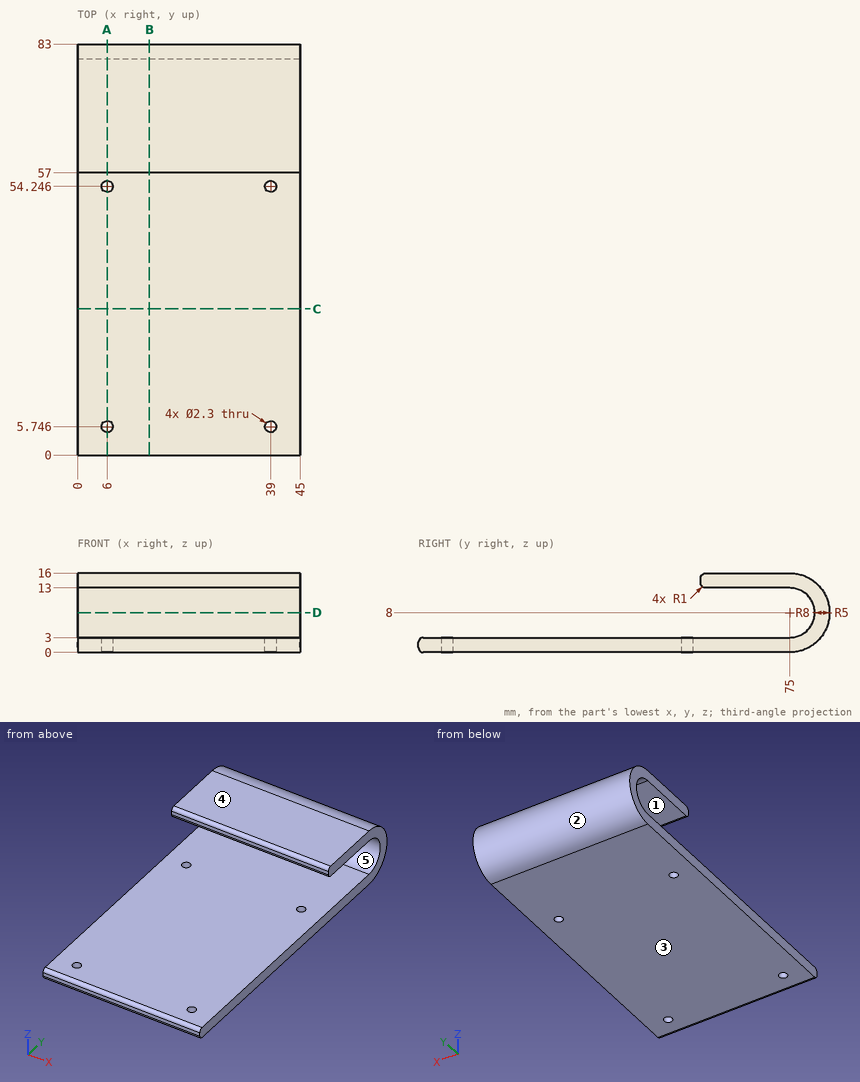
Can you work these out from the drawing? Everything is in mm from the part's minimum corner. A direction names the side the tool comes from. Coordinates: 2 decimals unless noted, no trailing zeros. Loops run counter-clockwise (first coordinate to the right, second up) from the corner with the lowest first, then second, coordinate; pieces in that order, holes last. Notation, with made-up numbers: (-38.75, 53) - (-31.75, 53) arc R11 ccw to (-31.75, 64) - close; hole circle Ø6 at (83, 40.5). An arc over 180 degrees is marked (long way). Use a Markdown table: item, result.
Item 1: I want a section at C-C on y = 29.5. Please give me the cut outline in (x, z), and give its area (3 significant figures).
Numbers:
| item | result |
|---|---|
| outline | (0, 0) - (45, 0) - (45, 3) - (0, 3) - close |
| area | 135 mm2 |
Item 2: I want a section at D-D on z = 8. Please give me the cut outline in (x, y), and give its area (3 significant figures).
Numbers:
| item | result |
|---|---|
| outline | (0, 80) - (45, 80) - (45, 83) - (0, 83) - close |
| area | 135 mm2 |
Item 3: I want a section at A-A on x = 6. Please give me the cut outline in (y, z), and give its area (3 significant figures).
Numbers:
| item | result |
|---|---|
| outline | (0, 1) arc R1 ccw to (1, 0) - (4.6, 0) - (4.6, 3) - (1, 3) arc R1 ccw to (0, 2) - close; (6.9, 0) - (53.1, 0) - (53.1, 3) - (6.9, 3) - close; (55.4, 0) - (75, 0) arc R8 ccw to (75, 16) - (58, 16) arc R1 ccw to (57, 15) - (57, 14) arc R1 ccw to (58, 13) - (75, 13) arc R5 cw to (75, 3) - (55.4, 3) - close |
| area | 326 mm2 |
Item 4: If I drill on probe 1 along Y at (x, z) = (6, 1.15) (1 decimal); probe 2 along Y at (x, z) = (39, 0.8) (1 decimal); probe 3 along Z at (x, y) = (28, 66.5), over which ranges is the centre line in solid material (lowest first)? Write a range as from..to.
Numbers:
| item | result |
|---|---|
| probe 1 | y = 0..4.6, 6.9..53.1, 55.4..79.1 |
| probe 2 | y = 0..4.6, 6.9..53.1, 55.4..78.5 |
| probe 3 | z = 0..3, 13..16 |
Item 5: For the marked faces 1 and 2, which set-ups out of +Z, -Z, +X, -X, +Y, -Y let a thin tool reach every point of the face, with its end or its side?
Numbers:
| item | result |
|---|---|
| face 1 | +X, -X, -Y |
| face 2 | +X, -X, +Y |
Item 6: We'd pull the mould along Z, two halves only. Please class the marked faces 3, 4 and 5: released by +Z, released by -Z, zero draft, split by the parting line, or undercut.
Numbers:
| item | result |
|---|---|
| face 3 | released by -Z |
| face 4 | released by +Z |
| face 5 | undercut |
Item 7: I want a section at B-B on x = 14.5. Please give me the cut outline in (y, z).
Numbers:
| item | result |
|---|---|
| outline | (0, 1) arc R1 ccw to (1, 0) - (75, 0) arc R8 ccw to (75, 16) - (58, 16) arc R1 ccw to (57, 15) - (57, 14) arc R1 ccw to (58, 13) - (75, 13) arc R5 cw to (75, 3) - (1, 3) arc R1 ccw to (0, 2) - close |
Item 8: Will these pins go through, and if not, where does the flat tip stop? pin 1 (1.5 mm diameter, centred on x = 19, z = 11, fed in from +Y); pin 2 (0.8 mm diameter, centred on x = 27, z = 14.5, fed in from -Y); pin 3 (2 mm diameter, centred on x = 18, y = 41, fed in from +Z).
Numbers:
| item | result |
|---|---|
| pin 1 | stops at y = 82.68 |
| pin 2 | stops at y = 57 |
| pin 3 | stops at z = 3 |
